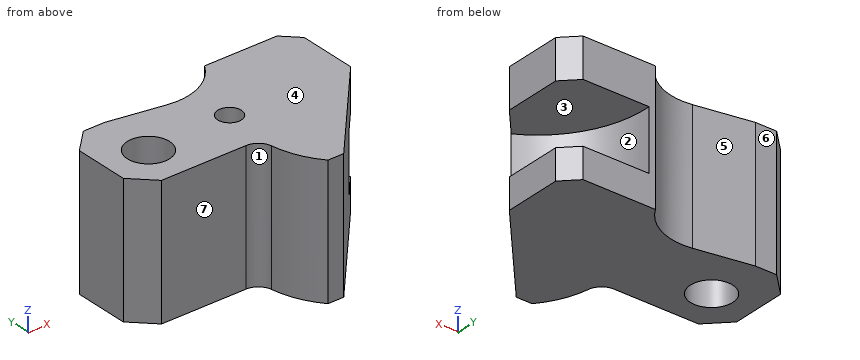
```python
from build123d import *

# Parameters (mm, degrees)
SKETCH1_R           = 7
BOSS_EXTRUDE1_DEPTH = 43
CUT_EXTRUDE1_START  = -10
SKETCH2_R           = 35.868634871
CUT_EXTRUDE1_DEPTH  = 20
SKETCH3_R           = 3.917707096
CUT_EXTRUDE2_DEPTH  = 23


with BuildPart() as part:
    # Sketch1 → Boss-Extrude1 (new body)
    with BuildSketch(Plane.XY):
        with BuildLine():
            Line((-14, -7), (-14, 11))
            Line((-14, 11), (-7, 18))
            Line((-7, 18), (0, 18))
            Line((0, 18), (18.243084988, 14.783251905))
            ThreePointArc((18.243084988, 14.783251905), (29.574972961, 16.276069151), (38, 24))
            Line((38, 24), (62, 24))
            Line((62, 24), (67, 19))
            Line((67, 19), (67, 0))
            Line((67, 0), (38, -33))
            Line((38, -33), (32.788067397, -33))
            ThreePointArc((32.788067397, -33), (28.3490952, -26.115672061), (26.012264997, -18.264705882))
            ThreePointArc((26.012264997, -18.264705882), (24.331862036, -15.213413768), (21.066626255, -14))
            Line((21.066626255, -14), (-7, -14))
            Line((-7, -14), (-14, -7))
        make_face()
        Circle(SKETCH1_R, mode=Mode.SUBTRACT)
    extrude(amount=BOSS_EXTRUDE1_DEPTH)

    # Sketch2 → Cut-Extrude1 (cut)
    with BuildSketch(Plane(origin=(0, 0, 0), x_dir=(-1, 0, 0), z_dir=(0, 0, -1)).offset(CUT_EXTRUDE1_START)):
        with Locations((-75.938611571, 22.638320419)):
            Circle(SKETCH2_R)
    extrude(amount=-CUT_EXTRUDE1_DEPTH, mode=Mode.SUBTRACT)

    # Sketch3 → Cut-Extrude2 (cut)
    with BuildSketch(Plane.XY.offset(43)):
        with Locations((27.374932955, 0.618357786)):
            Circle(SKETCH3_R)
    extrude(amount=-CUT_EXTRUDE2_DEPTH, mode=Mode.SUBTRACT)


solid = part.part
```
Model file for the job. Use its own axes, mm. Face numbers are marked on the shaded views. A direction names the side the tool comes from. Give positions to 0.01 mm unless a question says otherwise; leave off trailing zeros. Loops run counter-clockwise (first coordinate to the right, second up) from the corner with the lowest first, then second, coordinate; pieces in that order, holes last. Notation, with made-up numbers: (88, 79.25) -> (96, 79.25) arc R9 cw to (96, 94.25) -> close; hole circle Ø7 at (-40, 85). An arc over 180 degrees is marked (long way). Use CSV: the item, a comma, the result in double quotes. Start each with the question number.
1) Wall check: line 1 (Y direction, x = 0, z = 21); line 2 (Z direction, x = 46, y = 15); line 3 (X direction, y = 5.5, z = 37.5). Give the ranges that are in metal, low to high.
2) Slice it at C-C on z = 34.5. Give the cut face in (x, y), plus the area to 3 significant figures.
3) Slice it at B-B on x = -3. Give the cut face in (y, z), plus the area to 3 significant figures.
4) Mould opens along Z. For the marked faces 1, 2, 3 and 4 say: released by +Z, released by -Z, zero draft, split by the parting line, or undercut.
5) Slice it at A-A on z = 6. Give the cut face in (x, y).
6) Tool access for the marked faces 5, 6 and 7: list every direction of +Z, -Z, +X, -X, +Y, -Y with a clear straight run to the whole face (end or side of a thin tool).
7) Slice it at D-D on x = 58. Give the cut face in (y, z), plus the area to 3 significant figures.
8) Flat gauge pins, fed straight in: pin 1 Ø22.5 at (x, z) = (8, 28) entering from -Y; pin 2 Ø2 at (x, z) = (5.5, 22.5) entering from +Y; pin 3 Ø1.5 at (y, z) = (-22.5, 38) entering from -X; pin 4 Ø6.5 at (x, y) = (27.37, 0.62) entering from -Z. Where does each tip first touch, or does it go through?
Computed values:
1,line 1,"y = -14 to -7, 7 to 18"
1,line 2,"z = 0 to 10, 30 to 43"
1,line 3,"x = -14 to -4.33, 4.33 to 67"
2,outline,"(-14, -7) -> (-7, -14) -> (21.07, -14) arc R5 cw to (26.01, -18.26) arc R29 ccw to (32.79, -33) -> (38, -33) -> (67, 0) -> (67, 19) -> (62, 24) -> (38, 24) arc R19 cw to (18.24, 14.78) -> (0, 18) -> (-7, 18) -> (-14, 11) -> close; hole circle Ø14 at (0, 0); hole circle Ø7.84 at (27.37, 0.62)"
2,area,"2,720 mm^2"
3,outline,"(-14, 0) -> (-6.32, 0) -> (-6.32, 43) -> (-14, 43) -> close; (6.32, 0) -> (18, 0) -> (18, 43) -> (6.32, 43) -> close"
3,area,"832 mm^2"
4,face 1,"zero draft"
4,face 2,"undercut"
4,face 3,"undercut"
4,face 4,"released by +Z"
5,outline,"(-14, -7) -> (-7, -14) -> (21.07, -14) arc R5 cw to (26.01, -18.26) arc R29 ccw to (32.79, -33) -> (38, -33) -> (67, 0) -> (67, 19) -> (62, 24) -> (38, 24) arc R19 cw to (18.24, 14.78) -> (0, 18) -> (-7, 18) -> (-14, 11) -> close; hole circle Ø14 at (0, 0)"
6,face 5,"+Z, -Z, +Y"
6,face 6,"+Z, -Z, -X, +Y"
6,face 7,"+Z, -Z, -X, -Y"
7,outline,"(-10.24, 0) -> (24, 0) -> (24, 10) -> (-8.42, 10) -> (-8.42, 30) -> (24, 30) -> (24, 43) -> (-10.24, 43) -> close"
7,area,"824 mm^2"
8,pin 1,"stops at y = -14"
8,pin 2,"stops at y = 17.21"
8,pin 3,"stops at x = 26.75"
8,pin 4,"stops at z = 0"
